CAD build for the part. Positions are in the model's coordinates, mm. A direction names the side the tool comes from. Give positions to 0.01 mm unless a question says otherwise; leave off trailing zeros. Order: outer loops, then holes, each group sorted by start corner. A loop starts at its lowest first (then second) coordinate and runs counter-clockwise, first axis right, second up.
Autodesk Inventor part; units mm, degrees
ref_plane "COMBINATION_MODULE_XY" through (0, 0, 0) normal (1, 0, 0) x (0, 0, -1)
ref_plane "COMBINATION_MODULE_YZ" through (0, 0, 0) normal (0, 0, -1) x (0, 1, 0)
ref_plane "COMBINATION_MODULE_ZX" through (0, 0, 0) normal (0, 1, 0) x (1, 0, 0)
sketch "Sketch_1" plane through (0, 0, 0) normal (0, 0, 1) x (1, 0, 0)
  line L0 (68, 0) -> (0, 0)
  line L1 (0, 0) -> (0, 4.5)
  line L2 (0, 4.5) -> (0.5, 5)
  line L3 (0.5, 5) -> (67.5, 5)
  line L4 (67.5, 5) -> (68, 4.5)
  line L5 (68, 4.5) -> (68, 0)
  line L6 (68, 0) -> (0, 0)
revolve "Revolution1" add sketch "Sketch_1" angle 360 about axis through (68, 0, 0) along (1, 0, 0)
sketch "_____10" plane through (0, 0, 5) normal (0, 0, 1) x (1, 0, 0)
  arc A0 (33, 1.5) -> (33, -1.5) centre (33, 0) ccw
  line L0 (33, -1.5) -> (41, -1.5)
  arc A1 (41, -1.5) -> (41, 1.5) centre (41, 0) ccw
  line L1 (41, 1.5) -> (33, 1.5)
extrude "Extrusion1" cut sketch "_____10" against normal blind 1.8
sketch "_____5" plane through (3, 0, 0) normal (1, 0, 0) x (0, 0, -1)
  circle A0 centre (0, 0) radius 10
  circle A1 centre (0, 0) radius 4.8
extrude "Extrusion2" cut sketch "_____5" against normal blind 1.15
sketch "_____6" plane through (65, 0, 0) normal (1, 0, 0) x (0, 0, -1)
  circle A0 centre (0, 0) radius 10
  circle A1 centre (0, 0) radius 4.8
extrude "Extrusion3" cut sketch "_____6" along normal blind 1.15
ref_plane "COMBINATION_MODULE_XY" through (0, 0, 0) normal (1, 0, 0) x (0, 0, -1)
ref_plane "COMBINATION_MODULE_YZ" through (0, 0, 0) normal (0, 0, -1) x (0, 1, 0)
ref_plane "COMBINATION_MODULE_ZX" through (0, 0, 0) normal (0, 1, 0) x (1, 0, 0)
ref_plane "to_ring_b_XY" through (2.425, 0, 0) normal (1, 0, 0) x (0, 0, -1)
ref_plane "to_ring_b_YZ" through (2.425, 0, 0) normal (0, 0, -1) x (0, 1, 0)
ref_plane "to_ring_b_ZX" through (2.425, 0, 0) normal (0, 1, 0) x (1, 0, 0)
ref_plane "to_ring_s_XY" through (65.575, 0, 0) normal (1, 0, 0) x (0, 0, -1)
ref_plane "to_ring_s_YZ" through (65.575, 0, 0) normal (0, 0, -1) x (0, 1, 0)
ref_plane "to_ring_s_ZX" through (65.575, 0, 0) normal (0, 1, 0) x (1, 0, 0)
properties part number "NSFMRRA10-68-B3-S3-KC31.5-A11(000_000)_s"
1. Pin check, flat tips, straight feed: P1, Ø4, axis at x = 27, z = -4, coming from the +Y side; P2, Ø6, axis at x = 13, y = 4, coming from the +Z side; P3, Ø2.5, axis at x = 35, y = 0.5, coming from the +Z side. Stop position of each tip, or through.
2. Mould opens along Y. For faces 1 (the cylindrical face through (65.57, -4.05, -2.58)), 2 (the flat face through (68, 0, 0)), 3 (the flat face through (37, 1.5, 4)) say: released by +Y, released by -Y, zero draft, split by the parting line, or undercut.
3. 3-axis set-ups, long thin cutter, end or side, ignore diameter. For faces 4 (the cylindrical face through (2.43, 4.05, -2.58)), 5 (the flat face through (37, -1.5, 4)), 6 (the flat face through (0, 0, 0)): which of +Z, -Z, +X, -X, +Y, -Y reach the whole face in a straight line?
4. Saw through at B-B on x = 28.5. Give the cut face in (y, z), plus the area to 3 significant figures.
5. Wall check: line 1 (X direction, y = -0.75, z = 4.25); line 2 (Y direction, x = 61, z = 0.25); line 3 (Z direction, x = 15, y = 1.75). Give the ranges that are in metal, low to high.
6. Saw through at A-A on y = 0. Give the cut face in (x, z), plus the area to 3 significant figures.
7. Saw through at C-C on x = 36. Give the cut face in (y, z), plus the area to 3 significant figures.
Reported:
1. P1: stops at y = 4.58
1. P2: stops at z = 4.9
1. P3: stops at z = 4.77
2. face 1: split by the parting line
2. face 2: zero draft
2. face 3: undercut
3. face 4: none
3. face 5: +Z
3. face 6: +Z, -Z, -X, +Y, -Y
4. outline: circle Ø10 at (0, 0)
4. area: 78.5 mm2
5. line 1: x = 0 to 31.7, 42.3 to 68
5. line 2: y = -4.99 to 4.99
5. line 3: z = -4.68 to 4.68
6. outline: (0, -4.5) - (0.5, -5) - (1.85, -5) - (1.85, -4.8) - (3, -4.8) - (3, -5) - (65, -5) - (65, -4.8) - (66.15, -4.8) - (66.15, -5) - (67.5, -5) - (68, -4.5) - (68, 4.5) - (67.5, 5) - (66.15, 5) - (66.15, 4.8) - (65, 4.8) - (65, 5) - (42.5, 5) - (42.5, 3.2) - (31.5, 3.2) - (31.5, 5) - (3, 5) - (3, 4.8) - (1.85, 4.8) - (1.85, 5) - (0.5, 5) - (0, 4.5) - close
6. area: 659 mm2
7. outline: (-1.5, 3.2) - (-1.5, 4.77) arc R5 ccw (long way) to (1.5, 4.77) - (1.5, 3.2) - close
7. area: 73.4 mm2
